The model under review builds one solid part; all positions refer to its coordinate system, in mm. A direction names the side the tool comes from. Give positions to 0.01 mm unless a question says otherwise; leave off trailing zeros. Loops run counter-clockwise (first coordinate to the right, second up) from the corner with the lowest first, then second, coordinate; pieces in that order, holes last. Notation, with made-up numbers: M 71.5,-10 L 113.5,-10 A16 cw 113.5,13 Z; hole C 48.5,8.25 d3. An arc over 180 degrees is marked long. Put each result on its own line as item: value. Start each with the question number.
```python
from build123d import *

# Parameters (mm, degrees)
SALIENTE_EXTRUIR1_DEPTH       = 20
CROQUIS2_R                    = 14
CORTAR_EXTRUIR1_DEPTH         = 63.174085438
CHAFL_N1_SIZE                 = 0.5
TALADRO_ROSCADO_M5X0_81_D     = 4.2
TALADRO_ROSCADO_M5X0_81_DEPTH = 16
TALADRO_ROSCADO_M5X0_81_TIP   = 1.2618073


with BuildPart() as part:
    # Croquis1 → Saliente-Extruir1 (new, symmetric)
    with BuildSketch(Plane.XY):
        Polygon((26, 0), (-26, 0), (-26, 28.154625486), (-13, 39.87), (13, 39.87), (26, 28.154625486), align=None)
    extrude(amount=SALIENTE_EXTRUIR1_DEPTH, both=True)

    # Croquis2 → Cortar-Extruir1 (cut, through all)
    with BuildSketch(Plane.XY.offset(20)):
        with Locations((0, 20)):
            Circle(CROQUIS2_R)
    extrude(amount=-CORTAR_EXTRUIR1_DEPTH, mode=Mode.SUBTRACT)

    # Chaflán1
    chafl_n1_edges = [part.edges().sort_by_distance(p)[0] for p in [
        (-14, 20, -20),
        (-14, 20, 20),
    ]]
    chamfer(chafl_n1_edges, length=CHAFL_N1_SIZE)

    # Taladro roscado M5x0.81
    with Locations(Plane(origin=(0, 0, 0), x_dir=(-1, 0, 0), z_dir=(0, -1, 0))):
        with Locations((-20, -12), (20, -12), (20, 12), (-20, 12)):
            Hole(TALADRO_ROSCADO_M5X0_81_D / 2, depth=TALADRO_ROSCADO_M5X0_81_DEPTH)
            with Locations((0, 0, -(TALADRO_ROSCADO_M5X0_81_DEPTH + TALADRO_ROSCADO_M5X0_81_TIP / 2))):  # 118° drill point
                Cone(0, TALADRO_ROSCADO_M5X0_81_D / 2, TALADRO_ROSCADO_M5X0_81_TIP, mode=Mode.SUBTRACT)


solid = part.part
```
Item 1: Consider section C-C, the plane y = 9.5. Give the number of separate pieces and of enclosed holes in the cut face, plus the area to 3 significant figures.
Item 2: Clearance check with flat-ended pins moving along their axes: pin 1 Ø2 at (y, z) = (31, 6.5) entering from -X; pin 2 Ø5.5 at (x, z) = (-20, -12) entering from +Y. State where each tip first meets the part, or that it passes through.
Item 3: Consider section A-A, the plane y = 3. Write out the cut boundary in (x, z), plus the area to 3 significant figures.
Item 4: Draft analysis for pull direction Z (two halves, no side actions). For faces 1 (the flat face through (-26, 14, 0)), 2 (the cylindrical face through (22.003, 8.112, 11.369)), 3 (the flat face through (12, 11, -20)), state which applies: +Z half, -Z half, draft (parallel to the pull), parting line (faces both ways), or undercut.
Item 5: To check wall thickness, follow L1, parallel to Y at x = 0, z = -10; L2, parallel to Z at x = -20, y = 8; L3, parallel to Z at x = -19, y = 6.5. State the ranges of each line that lie inside material, in increasing order. Write a range as [from, to].
Item 6: Consider section B-B, the plane z = 6.5. Write out the cut boundary in (x, y).
Item 7: Consider section D-D, the plane x = -17. Write out the cut boundary in (y, z).
Item 8: Tool access review of faces 4 (the flat face through (0, 39.87, 0)), 5 (the cylindrical face through (-17.997, 8.112, 11.369)): name each direction out of +Z, -Z, +X, -X, +Y, -Y from which nothing blocks a thin tool from reaching the whole face with its end or side.
Report:
1. separate pieces: 2
1. enclosed holes: 4
1. area: 1,280 mm²
2. pin 1: x = -23.95
2. pin 2: y = 36.04
3. outline: M -26,-20 L 26,-20 L 26,20 L -26,20 Z; hole C -20,-12 d4.2; hole C -20,12 d4.2; hole C 20,-12 d4.2; hole C 20,12 d4.2
3. area: 2,020 mm²
4. face 1: draft
4. face 2: undercut
4. face 3: -Z half
5. L1: [0, 6], [34, 39.87]
5. L2: [-20, -14.1], [-9.9, 9.9], [14.1, 20]
5. L3: [-20, -13.85], [-10.15, 10.15], [13.85, 20]
6. outline: M -26,0 L 26,0 L 26,28.15 L 13,39.87 L -13,39.87 L -26,28.15 Z; hole C 0,20 d28
7. outline: M 0,-20 L 36.27,-20 L 36.27,20 L 0,20 Z
8. face 4: +Z, -Z, +X, -X, +Y
8. face 5: -Y
